Verification items for this drawing (mm, ordinates from the low corner). Coordinates: 2 decimals unless noted, no trailing zeros. Write each loop counter-clockwise with the first axis right and the second up, starting at its lowest first coordinate (ties: lowest second). Pieces come first, ordered by that corner, then holes. Notation, with made-up numbers: (10, 88) -> (66, 88) arc R18 ccw to (66, 95) -> close; hole circle Ø10 at (75.5, 71). An arc over 180 degrees is marked (long way). Put each result on its own line as item: value. Start each with the question number.
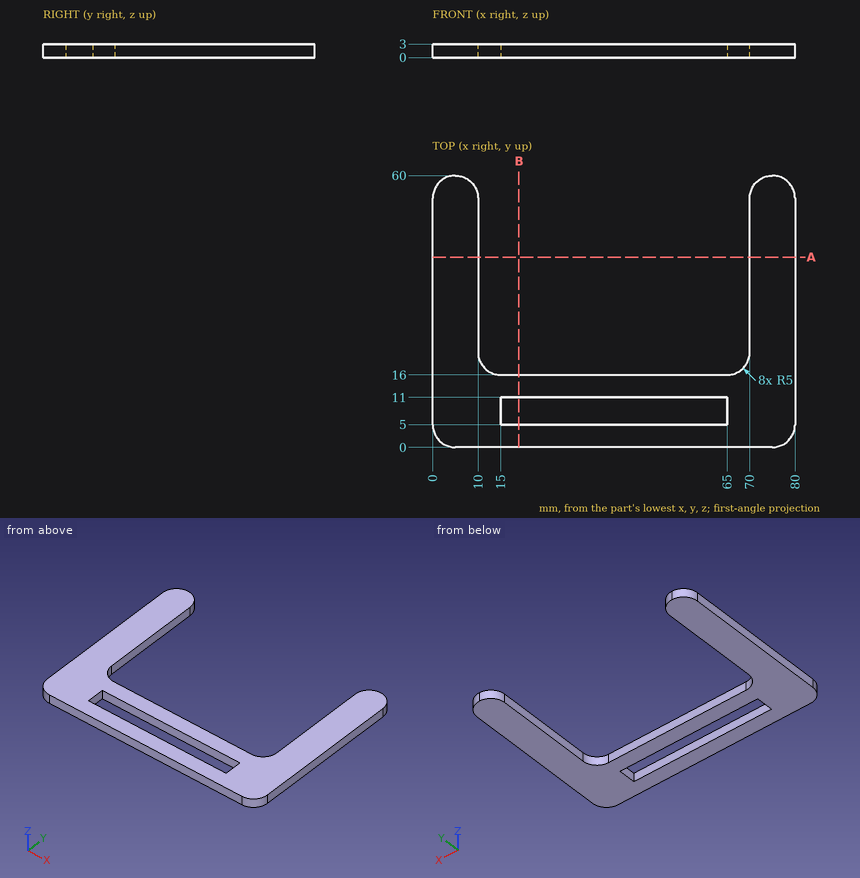
Item 1: Section check A-A, the plane y = 42. Enter the section's corners in (x, z).
Item 2: Go/stop test with flat-tipped pins: P1, Ø1, axis at x = 67.5, z = 2, coming from the +Y side; P2, Ø0.9, axis at y = 31.5, z = 1.5, coming from the -X side; P3, Ø1, axis at x = 11, z = 1, coming from the +Y side. Record where each tip stops, or that it passes through.
Item 3: Scan lines: line 1 along Y through (x, z) = (32, 2.45); line 2 along X through (y, z) = (52, 1.3); line 3 along X through (y, z) = (17, 2). Record each from-to range of solid material in increasing order. Write a range as [from, to].
Item 4: Section check B-B, the plane x = 19. Enter the section's corners in (y, z).
From the geometry:
1. outline: (0, 0) -> (10, 0) -> (10, 3) -> (0, 3) -> close; (70, 0) -> (80, 0) -> (80, 3) -> (70, 3) -> close
2. P1: y = 17
2. P2: x = 0
2. P3: y = 18.82
3. line 1: [0, 5], [11, 16]
3. line 2: [0, 10], [70, 80]
3. line 3: [0, 12], [68, 80]
4. outline: (0, 0) -> (5, 0) -> (5, 3) -> (0, 3) -> close; (11, 0) -> (16, 0) -> (16, 3) -> (11, 3) -> close
